from build123d import *

# Parameters (mm, degrees)
EXTRUDE_1_DEPTH = 40


with BuildPart() as part:
    # Эскиз1 → Бобышка-Вытянуть1 (new body)
    with BuildSketch(Plane.XY):
        with BuildLine():
            Line((0, 25.8), (0, 24.3))
            ThreePointArc((0, 24.3), (12.712002203, 20.709780298), (21.667717923, 11))
            Line((21.667717923, 11), (23.337523433, 11))
            ThreePointArc((23.337523433, 11), (13.81738036, 21.78807013), (0, 25.8))
        make_face()
        with BuildLine():
            ThreePointArc((24.217555616, 2), (-16.460407042, -17.875821659), (0, 24.3))
            Line((0, 24.3), (0, 25.8))
            ThreePointArc((0, 25.8), (-17.521986189, -18.93726485), (25.722363811, 2))
            Line((25.722363811, 2), (24.217555616, 2))
        make_face()
    extrude(amount=EXTRUDE_1_DEPTH)


solid = part.part
Input: part model. Units: mm. Frame: model coordinates. A direction names the side the tool comes from. Coordinates: 2 decimals unless noted, no trailing zeros. Loops run counter-clockwise (first coordinate to the right, second up) from the corner with the lowest first, then second, coordinate; pieces in that order, holes last.
(1) First-contact query: pin 1 Ø1 at (y, z) = (15.5, 14.5) entering from -X; pin 2 Ø0.5 at (x, z) = (25, 19.5) entering from +Y; pin 3 Ø3 at (y, z) = (-20, 7) entering from +X. Flat tips, straight axial feed; report the tip coordinate or a pass-through.
(2) Section A-A on y = 0. Return the cut outline in (x, z), then the cut area to 3 significant figures.
(3) Material intervals for probe 1 along Y at (x, z) = (0, 11.5); probe 2 along Y at (x, z) = (-12, 4), sorted ascending.
(4) Set-up query: faces 1 (the face through (25, 2, 20)), 2 (the face through (-19.2, -15.2, 40)), 3 (the face through (22, 11, 20)). Return all of +Z, -Z, +X, -X, +Y, -Y with unobstructed straight access to the full face (end or side cutting, diameter ignored); none if empty.
(5) Section C-C on z = 36. Return the cut outline in (x, y), then the cut area to 3 significant figures.
(6) Section B-B on x = -1.5. Return the cut outline in (y, z), then the cut area to 3 significant figures.
Data:
1. pin 1: stops at x = -20.99
1. pin 2: stops at y = 2
1. pin 3: stops at x = 17.98
2. outline: (-25.8, 0) - (-24.3, 0) - (-24.3, 40) - (-25.8, 40) - close; (24.3, 0) - (25.8, 0) - (25.8, 40) - (24.3, 40) - close
2. area: 120 mm2
3. probe 1: y = -25.8 to -24.3, 24.3 to 25.8
3. probe 2: y = -22.84 to -21.13, 21.13 to 22.84
4. face 1: +Z, -Z, +X, +Y
4. face 2: +Z, +X, -X, +Y, -Y
4. face 3: +Z, -Z, +X
5. outline: (21.67, 11) - (23.34, 11) arc R25.8 ccw (long way) to (25.72, 2) - (24.22, 2) arc R24.3 cw (long way) to start
5. area: 222 mm2
6. outline: (-25.76, 0) - (-24.25, 0) - (-24.25, 40) - (-25.76, 40) - close; (24.25, 0) - (25.76, 0) - (25.76, 40) - (24.25, 40) - close
6. area: 120 mm2
